Build history of the part. All positions in model axes, mm. A direction names the side the tool comes from. Give positions to 0.01 mm unless a question says otherwise; leave off trailing zeros. Loops run counter-clockwise (first coordinate to the right, second up) from the corner with the lowest first, then second, coordinate; pieces in that order, holes last. Notation, with made-up numbers: (-12, -20.5) - (45, -20.5) arc R18 ccw to (45, -7.5) - close; hole circle Ø5 at (60, 66). An arc over 180 degrees is marked (long way). Return JSON: item names as keys, results as strings. Group by question number.
1) Slice it at B-B (y = 6.25). List the corners of the cut face in (x, z).
2) Mould opens along Y. For faces 3 (the face through (5, -10, 0)), 4 (the face through (-0.96, -10.64, 1.82)), 5 (the face through (11.923, 3.755, 1.825)) say: released by +Y, released by -Y, zero draft, split by the parting line, or undercut.
3) Drill centre lines: probe 1 along Y at (x, z) = (0, 0.95); probe 2 along X at (y, z) = (-4.5, 2.4); probe 3 along X at (y, z) = (1.75, 2.15). Where is each one in solid material? Low to high. Write a range as from..to.
4) Slice it at C-C (z = 2.6). Count the separate pieces of the cut face and the enclosed holes in it, and give its area (3 significant figures).
5) Drop flat-ended pins along their axis: pin 1 (3 mm diameter, centred on x = 1, y = 7.5, fed in from +Z); pin 2 (0.6 mm diameter, centred on y = -9.5, z = 2.5, fed in from +X); pin 3 (2 mm diameter, centred on y = -1.5, z = 1.5, fed in from +X). Give the stop position or say it passes through.
6) Slice it at A-A (x = 0). List the corners of the cut face in (y, z), and give its area (3 significant figures).
7) 3-axis set-ups, long thin cutter, end or side, ignore diameter. For faces 1 (the face through (-0.842, 8.712, 1.779)), 2 (the face through (-5, 6, 3.3)): which of +Z, -Z, +X, -X, +Y, -Y reach the whole face in a straight line?
```python
from build123d import *

# Parameters (mm, degrees)
SKETCH_1_R          = 8.5
SKETCH_1_R_2        = 7.5
EXTRUDE_1_DEPTH     = 3.6
SKETCH_2_R          = 12.5
SKETCH_2_R_2        = 11
EXTRUDE_2_DEPTH     = 3.6
EXTRUDE_START       = -3
EXTRUDE_3_DEPTH     = 3
FILLET_1_R          = 1
CUT_EXTRUDE_START   = -0.3
SKETCH_5_R          = 8.5
SKETCH_5_R_2        = 7.5
CUT_EXTRUDE_1_DEPTH = 0.3
SKETCH_6_R          = 8.5
SKETCH_6_R_2        = 7.5
CUT_EXTRUDE_2_DEPTH = 0.3


with BuildPart() as part:
    # Sketch 1 → Extrude 1 (new body)
    with BuildSketch(Plane.XY):
        Circle(SKETCH_1_R)
        Circle(SKETCH_1_R_2, mode=Mode.SUBTRACT)
    extrude(amount=EXTRUDE_1_DEPTH)



with BuildPart() as body_2:
    # Sketch 2 → Extrude 2 (new body)
    with BuildSketch(Plane.XY.offset(3.6)):
        Circle(SKETCH_2_R)
        Circle(SKETCH_2_R_2, mode=Mode.SUBTRACT)
    extrude(amount=-EXTRUDE_2_DEPTH)


with BuildPart() as part_1:
    add(part.part)

    add(body_2.part)  # Extrude 3 merges body 2
    # Sketch 4 → Extrude 3 (add)
    with BuildSketch(Plane.XY.offset(3.3).offset(EXTRUDE_START)):
        with BuildLine():
            ThreePointArc((-0.6, 8.478797084), (0, 8.5), (0.6, 8.478797084))
            Line((0.6, 8.478797084), (0.6, 10.983624174))
            ThreePointArc((0.6, 10.983624174), (0, 11), (-0.6, 10.983624174))
            Line((-0.6, 10.983624174), (-0.6, 8.478797084))
        make_face()
        with BuildLine():
            Line((-11, 0), (-8.5, 0))
            ThreePointArc((-8.5, 0), (-8.494697617, 0.30018726), (-8.478797084, 0.6))
            Line((-8.478797084, 0.6), (-10.983624174, 0.6))
            ThreePointArc((-10.983624174, 0.6), (-10.995905281, 0.300111716), (-11, 0))
        make_face()
        with BuildLine():
            Line((0.6, -10.983624174), (0.6, -8.478797084))
            ThreePointArc((0.6, -8.478797084), (0, -8.5), (-0.6, -8.478797084))
            Line((-0.6, -8.478797084), (-0.6, -10.983624174))
            ThreePointArc((-0.6, -10.983624174), (0, -11), (0.6, -10.983624174))
        make_face()
        with BuildLine():
            ThreePointArc((8.478797084, 0.6), (8.494697617, 0.30018726), (8.5, 0))
            Line((8.5, 0), (11, 0))
            ThreePointArc((11, 0), (10.995905281, 0.300111716), (10.983624174, 0.6))
            Line((10.983624174, 0.6), (8.478797084, 0.6))
        make_face()
        with BuildLine():
            Line((8, 0), (8.5, 0))
            ThreePointArc((8.5, 0), (8.494697617, 0.30018726), (8.478797084, 0.6))
            Line((8.478797084, 0.6), (8, 0.6))
            Line((8, 0.6), (8, 0))
        make_face()
        with BuildLine():
            ThreePointArc((10.983624174, 0.6), (10.995905281, 0.300111716), (11, 0))
            ThreePointArc((11, 0), (10.995905281, -0.300111716), (10.983624174, -0.6))
            Line((10.983624174, -0.6), (11.5, -0.6))
            Line((11.5, -0.6), (11.5, 0.6))
            Line((11.5, 0.6), (10.983624174, 0.6))
        make_face()
        with BuildLine():
            Line((11, 0), (8.5, 0))
            ThreePointArc((8.5, 0), (8.494697617, -0.30018726), (8.478797084, -0.6))
            Line((8.478797084, -0.6), (10.983624174, -0.6))
            ThreePointArc((10.983624174, -0.6), (10.995905281, -0.300111716), (11, 0))
        make_face()
        with BuildLine():
            ThreePointArc((8.478797084, -0.6), (8.494697617, -0.30018726), (8.5, 0))
            Line((8.5, 0), (8, 0))
            Line((8, 0), (8, -0.6))
            Line((8, -0.6), (8.478797084, -0.6))
        make_face()
        with BuildLine():
            Line((0.6, -11.5), (0.6, -10.983624174))
            ThreePointArc((0.6, -10.983624174), (0, -11), (-0.6, -10.983624174))
            Line((-0.6, -10.983624174), (-0.6, -11.5))
            Line((-0.6, -11.5), (0.6, -11.5))
        make_face()
        with BuildLine():
            ThreePointArc((-0.6, -8.478797084), (0, -8.5), (0.6, -8.478797084))
            Line((0.6, -8.478797084), (0.6, -8))
            Line((0.6, -8), (-0.6, -8))
            Line((-0.6, -8), (-0.6, -8.478797084))
        make_face()
        with BuildLine():
            ThreePointArc((-10.983624174, -0.6), (-10.995905281, -0.300111716), (-11, 0))
            ThreePointArc((-11, 0), (-10.995905281, 0.300111716), (-10.983624174, 0.6))
            Line((-10.983624174, 0.6), (-11.5, 0.6))
            Line((-11.5, 0.6), (-11.5, -0.6))
            Line((-11.5, -0.6), (-10.983624174, -0.6))
        make_face()
        with BuildLine():
            ThreePointArc((-8.478797084, -0.6), (-8.494697617, -0.30018726), (-8.5, 0))
            Line((-8.5, 0), (-11, 0))
            ThreePointArc((-11, 0), (-10.995905281, -0.300111716), (-10.983624174, -0.6))
            Line((-10.983624174, -0.6), (-8.478797084, -0.6))
        make_face()
        with BuildLine():
            Line((-8, -0.6), (-8, 0))
            Line((-8, 0), (-8.5, 0))
            ThreePointArc((-8.5, 0), (-8.494697617, -0.30018726), (-8.478797084, -0.6))
            Line((-8.478797084, -0.6), (-8, -0.6))
        make_face()
        with BuildLine():
            Line((-8.5, 0), (-8, 0))
            Line((-8, 0), (-8, 0.6))
            Line((-8, 0.6), (-8.478797084, 0.6))
            ThreePointArc((-8.478797084, 0.6), (-8.494697617, 0.30018726), (-8.5, 0))
        make_face()
        with BuildLine():
            ThreePointArc((-0.6, 10.983624174), (0, 11), (0.6, 10.983624174))
            Line((0.6, 10.983624174), (0.6, 11.5))
            Line((0.6, 11.5), (-0.6, 11.5))
            Line((-0.6, 11.5), (-0.6, 10.983624174))
        make_face()
        with BuildLine():
            Line((0.6, 8), (0.6, 8.478797084))
            ThreePointArc((0.6, 8.478797084), (0, 8.5), (-0.6, 8.478797084))
            Line((-0.6, 8.478797084), (-0.6, 8))
            Line((-0.6, 8), (0.6, 8))
        make_face()
    extrude(amount=EXTRUDE_3_DEPTH)

    # Fillet 1
    fillet_1_edges = [part_1.edges().sort_by_distance(p)[0] for p in [
        (0.6, 10.983624174, 1.8),
        (0.6, 8.478797084, 1.8),
        (-0.6, 8.478797084, 1.8),
        (8.478797084, -0.6, 1.8),
        (8.478797084, 0.6, 1.8),
        (10.983624174, 0.6, 1.8),
        (10.983624174, -0.6, 1.8),
        (0.6, -10.983624174, 1.8),
        (-0.6, -10.983624174, 1.8),
        (-0.6, -8.478797084, 1.8),
        (0.6, -8.478797084, 1.8),
        (-10.983624174, -0.6, 1.8),
        (-10.983624174, 0.6, 1.8),
        (-8.478797084, 0.6, 1.8),
        (-8.478797084, -0.6, 1.8),
        (-0.6, 10.983624174, 1.8),
    ]]
    fillet(fillet_1_edges, radius=FILLET_1_R)

    # Sketch 5 → Cut-Extrude 1 (cut)
    with BuildSketch(Plane.XY.offset(3.6).offset(CUT_EXTRUDE_START)):
        with Locations(Location((0, 0, 0), (0, 0, 170.303971602))):
            Circle(SKETCH_5_R)
        Circle(SKETCH_5_R_2, mode=Mode.SUBTRACT)
    extrude(amount=CUT_EXTRUDE_1_DEPTH, mode=Mode.SUBTRACT)

    # Sketch 6 → Cut-Extrude 2 (cut)
    with BuildSketch(Plane(origin=(0, 0, 0), x_dir=(-1, 0, 0), z_dir=(0, 0, -1))):
        Circle(SKETCH_6_R)
        Circle(SKETCH_6_R_2, mode=Mode.SUBTRACT)
    extrude(amount=-CUT_EXTRUDE_2_DEPTH, mode=Mode.SUBTRACT)


solid = part_1.part
```
Results:
{
 "1": {"outline": "(-10.83, 0) - (-9.05, 0) - (-9.05, 3.6) - (-10.83, 3.6) - close; (-5.76, 0.3) - (-4.15, 0.3) - (-4.15, 3.3) - (-5.76, 3.3) - close; (4.15, 0.3) - (5.76, 0.3) - (5.76, 3.3) - (4.15, 3.3) - close; (9.05, 0) - (10.83, 0) - (10.83, 3.6) - (9.05, 3.6) - close"},
 "2": {"face 3": "zero draft", "face 4": "undercut", "face 5": "split by the parting line"},
 "3": {"probe 1": "-12.5..-7.5, 7.5..12.5", "probe 2": "-11.66..-10.04, -7.21..-6, 6..7.21, 10.04..11.66", "probe 3": "-12.38..-10.86, -8.32..-7.29, 7.29..8.32, 10.86..12.38"},
 "4": {"separate pieces": "1", "enclosed holes": "5", "area": "177 mm2"},
 "5": {"pin 1": "z = 3.3", "pin 2": "x = 8.46", "pin 3": "x = 12.49"},
 "6": {"outline": "(-12.5, 0) - (-11, 0) - (-11, 0.3) - (-7.5, 0.3) - (-7.5, 3.3) - (-11, 3.3) - (-11, 3.6) - (-12.5, 3.6) - close; (7.5, 0.3) - (11, 0.3) - (11, 0) - (12.5, 0) - (12.5, 3.6) - (11, 3.6) - (11, 3.3) - (7.5, 3.3) - close", "area": "31.8 mm2"},
 "7": {"face 1": "+Z, -Z", "face 2": "+Z"}
}
